from build123d import *

# Parameters (mm, degrees)
F0_R     = 2.77
F0_R_2   = 2.5
F1_DEPTH = 0.97
F2_DEPTH = 8.6
F3_R     = 2.5
F4_W     = 0.2
F4_H     = 0.418926
F5_DEPTH = 2


with BuildPart() as f1:
    # F0 (on Top) → F1 (new body)
    with BuildSketch(Plane.XY):
        Circle(F0_R)
        Circle(F0_R_2, mode=Mode.SUBTRACT)
        Circle(F0_R_2)
    extrude(amount=F1_DEPTH)

    # F0 (on Top) → F2 (join)
    with BuildSketch(Plane.XY):
        Circle(F0_R_2)
    extrude(amount=F2_DEPTH)

    # F3
    f3_edges = [f1.edges().sort_by_distance(p)[0] for p in [
        (-2.5, 0, 8.6),
    ]]
    fillet(f3_edges, radius=F3_R)

    # F4 (on face) → F5 (join)
    with BuildSketch(Plane(origin=(0, 0, 0), x_dir=(1, 0, 0), z_dir=(0, 0, -1))):
        with Locations((-1.1, 0)):
            Rectangle(F4_W, F4_H)
        with Locations((1.1, 0)):
            Rectangle(F4_W, F4_H)
    extrude(amount=F5_DEPTH)


solid = f1.part
Can you work these out from the model? Positions are in its coordinate system, mm. A direction names the side the tool comes from. Coordinates: 2 decimals unless noted, no trailing zeros. Order: outer loops, then holes, each group sorted by start corner. A loop starts at its lowest first (then second) coordinate and runs counter-clockwise, first axis right, second up. Notation, with made-up numbers: (-29.5, -21) - (-22.5, -21) arc R9 ccw to (-22.5, -10) - close; hole circle Ø11 at (36.5, 77). An arc over 180 degrees is marked (long way). Answer as a JSON object with one key per item and string values. Group by question number.
Q1. Imagine slicing it at B-B (x = 0). Please give me the cut outline in (y, z).
Q2. Imagine slicing it at D-D (y = -0.75). Please give me the cut outline in (x, z).
Q3. Imagine slicing it at C-C (z = 5.75). Please give me the cut outline in (x, y), and give its area (3 significant figures).
Q4. I need wall thicknesses on line 1 (Z direction, x = 0.65, y = 2.5); line 2 (Z direction, x = 2.2, y = -0.3); line 3 (Y direction, x = 1, z = 8). Which ranges of each line are inside material? Lowest first, please. Write a range as from..to.
Q5. Imagine slicing it at A-A (y = 0). Please give me the cut outline in (x, z), and give its area (3 significant figures).
Q6. On a 3-axis mill with a long thin cutter (end or side, diameter ignored), from which of +Z, -Z, +X, -X, +Y, -Y can I reach the whole of each face in a straight line? I mean faces 1 (the face through (2.642, 0.832, 0.478)), 2 (the face through (-0.54, -2.44, 3.5)). Say none if no direction works.
Q7. Will these pins go through, and if not, where does the flat tip stop? P1, Ø1, axis at x = 0, z = 6.5, coming from the +Y side; P2, Ø1, axis at y = 2, z = 5.5, coming from the -X side; P3, Ø1.5, axis at y = -2, z = 0.5, coming from the +X side.
Determined:
{
 "1": {"outline": "(-2.77, 0) - (2.77, 0) - (2.77, 0.97) - (2.5, 0.97) - (2.5, 6.1) arc R2.5 ccw to (-2.5, 6.1) - (-2.5, 0.97) - (-2.77, 0.97) - close"},
 "2": {"outline": "(-2.67, 0) - (2.67, 0) - (2.67, 0.97) - (2.38, 0.97) - (2.38, 6.1) arc R2.38 ccw to (-2.38, 6.1) - (-2.38, 0.97) - (-2.67, 0.97) - close"},
 "3": {"outline": "circle Ø5 at (0, 0)", "area": "19.6 mm2"},
 "4": {"line 1": "z = 0..0.97", "line 2": "z = 0..7.25", "line 3": "y = -1.28..1.28"},
 "5": {"outline": "(-2.77, 0) - (-1.2, 0) - (-1.2, -2) - (-1, -2) - (-1, 0) - (1, 0) - (1, -2) - (1.2, -2) - (1.2, 0) - (2.77, 0) - (2.77, 0.97) - (2.5, 0.97) - (2.5, 6.1) arc R2.5 ccw to (-2.5, 6.1) - (-2.5, 0.97) - (-2.77, 0.97) - close", "area": "41.6 mm2"},
 "6": {"face 1": "+Z, -Z", "face 2": "+Z"},
 "7": {"P1": "stops at y = 2.5", "P2": "stops at x = -2", "P3": "stops at x = 2.47"}
}
